Design review of the part built by this model. Coordinates are the model's own, in mm. Face numbers are marked on the shaded views. Coordinates: 2 decimals unless noted, no trailing zeros. Order: outer loops, then holes, each group sorted by start corner. A loop starts at its lowest first (then second) coordinate and runs counter-clockwise, first axis right, second up. Notation, with made-up numbers: (19, -1.5) -> (25, -1.5) arc R22 cw to (25, 24.5) -> close; hole circle Ø5 at (77.25, -39). An arc over 180 degrees is marked (long way). Write item = value, one per line.
```python
from build123d import *

# Parameters (mm, degrees)
F0_R     = 63.5
F0_R_2   = 4.1275
F1_DEPTH = 25.4
F2_R     = 2.54
F3_R     = 9.7155
F4_DEPTH = 406.4


with BuildPart() as f1:
    # F0 (on Top) → F1 (new body)
    with BuildSketch(Plane.XY):
        Circle(F0_R)
        Circle(F0_R_2, mode=Mode.SUBTRACT)
    extrude(amount=F1_DEPTH)

    # F2
    f2_edges = [f1.edges().sort_by_distance(p)[0] for p in [
        (-63.5, 0, 25.4),
        (-63.5, 0, 0),
    ]]
    fillet(f2_edges, radius=F2_R)

    # F3 (on Top) → F4 (cut, symmetric)
    with BuildSketch(Plane.XY):
        Circle(F3_R)
    extrude(amount=F4_DEPTH, both=True, mode=Mode.SUBTRACT)


solid = f1.part
```
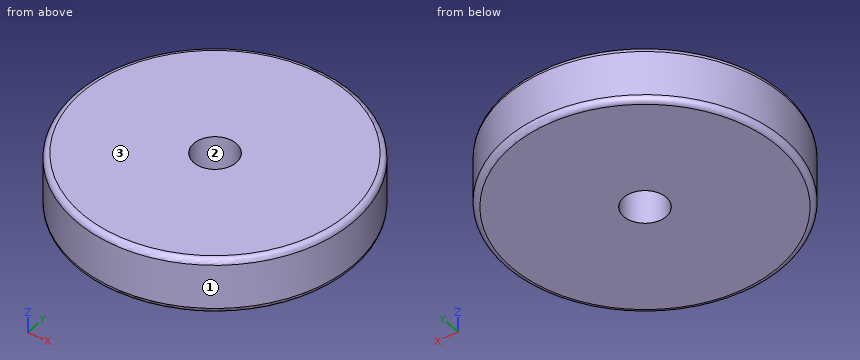
(1) The part is to be moulded in two halves that separate along Y. For the marked faces 1, 2 and 3, say which applies: released by +Y, released by -Y, zero draft, split by the parting line, or undercut.
Report:
face_1 = split by the parting line
face_2 = undercut
face_3 = zero draft
(2) Insertion check: pin 1 (8 mm diameter, centred on y = 37, z = 8.5, fed in from +X); pin 2 (1.5 mm diameter, centred on y = -10, z = 17, fed in from -X); pin 3 (3 mm diameter, centred on x = 35.5, z = 10, fed in from -Y). Each pin has a flat end and moves straight along its axis. Give the tip position at first contact, or say it passes through.
Report:
pin_1 = 54.25
pin_2 = -62.82
pin_3 = -53.63
(3) We need section A-A (y = 0). Write out the cut boundary in (x, z).
Report:
outline = (-63.5, 2.54) arc R2.54 ccw to (-60.96, 0) -> (-9.72, 0) -> (-9.72, 25.4) -> (-60.96, 25.4) arc R2.54 ccw to (-63.5, 22.86) -> close; (9.72, 0) -> (60.96, 0) arc R2.54 ccw to (63.5, 2.54) -> (63.5, 22.86) arc R2.54 ccw to (60.96, 25.4) -> (9.72, 25.4) -> close
(4) We need section C-C (z = 14.5). Write out the cut boundary in (x, y).
Report:
outline = circle Ø127 at (0, 0); hole circle Ø19.43 at (0, 0)
(5) For L1, parallel to Y at x = 0, z = 12.25; L2, parallel to Y at x = 8.5, z = 9; L3, parallel to X at y = -0.5, z = 1.5, list the stretches that pass through material, from the lowest coordinate up.
Report:
L1 = -63.5 to -9.72, 9.72 to 63.5
L2 = -62.93 to -4.71, 4.71 to 62.93
L3 = -63.28 to -9.7, 9.7 to 63.28
